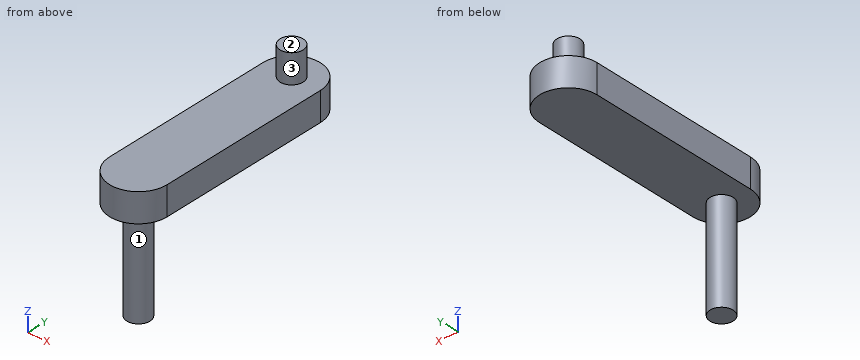
```python
from build123d import *

# Parameters (mm, degrees)
SKETCH1_R           = 4
BOSS_EXTRUDE1_DEPTH = 10
SKETCH1_2_R         = 4
BOSS_EXTRUDE2_DEPTH = 20
BOSS_EXTRUDE3_START = -35
SKETCH1_3_R         = 4
BOSS_EXTRUDE3_DEPTH = 45


with BuildPart() as part:
    # Sketch1 → Boss-Extrude1 (new body)
    with BuildSketch(Plane.XY):
        with BuildLine():
            Line((10, 30), (10, -30))
            ThreePointArc((10, -30), (0, -40), (-10, -30))
            Line((-10, -30), (-10, 30))
            ThreePointArc((-10, 30), (0, 40), (10, 30))
        make_face()
        with Locations((0, 30)):
            Circle(SKETCH1_R, mode=Mode.SUBTRACT)
        with Locations((0, -30)):
            Circle(SKETCH1_R, mode=Mode.SUBTRACT)
    extrude(amount=BOSS_EXTRUDE1_DEPTH)

    # Sketch1<2> → Boss-Extrude2 (add)
    with BuildSketch(Plane.XY):
        with Locations((0, 30)):
            Circle(SKETCH1_2_R)
    extrude(amount=BOSS_EXTRUDE2_DEPTH)

    # Sketch1<3> → Boss-Extrude3 (add)
    with BuildSketch(Plane.XY.offset(BOSS_EXTRUDE3_START)):
        with Locations((0, -30)):
            Circle(SKETCH1_3_R)
    extrude(amount=BOSS_EXTRUDE3_DEPTH)


solid = part.part
```
Geometry: final body of the model. Coordinates: model frame, mm. Face numbers are marked on the shaded views. A direction names the side the tool comes from. Coordinates: 2 decimals unless noted, no trailing zeros. Order: outer loops, then holes, each group sorted by start corner. A loop starts at its lowest first (then second) coordinate and runs counter-clockwise, first axis right, second up. Notation, with made-up numbers: M -3.5,-36 L 19.5,-36 A19 ccw 19.5,-14 Z; hole C 84.5,-33.75 d11. An arc over 180 degrees is marked long. Answer in a Markdown table with one row per item. Add a question column.
Q1. Section query A-A on x = 0. Return the cut outline in (y, z).
Q2. Line query: L1, parallel to Z at x = -2.75, y = -15.5; L2, parallel to Y at x = -0.25, z = -31.5; L3, parallel to X at y = -32, z = -16. Output: solid intervals per line, ascending.
Q3. Section query B-B on z = 14. Return the cut outline in (x, y).
Q4. Section query C-C on y = -13.5. Return the cut outline in (x, z), and give its area (3 significant figures).
Q5. Section query D-D on z = 3. Return the cut outline in (x, y).
Q6. Reachability of the marked faces 1, 2 and 3 from +Z, -Z, +X, -X, +Y, -Y: full face, straight path, thin tool, end or side. Return the list, or none.
Q7. Contact query for flat-ended pins moving along their axis: P1, Ø6, axis at x = 5, y = 10.5, coming from the +Z side; P2, Ø6, axis at x = 3.5, z = -19.5, coming from the +Y side; P3, Ø12, axis at x = 6.5, y = -12, coming from the -Z side. Output: stop coordinate, or through.
Completed:
| question | item | result |
|---|---|---|
| 1 | outline | M -40,0 L -34,0 L -34,-35 L -26,-35 L -26,0 L 40,0 L 40,10 L 34,10 L 34,20 L 26,20 L 26,10 L -40,10 Z |
| 2 | L1 | z = 0 to 10 |
| 2 | L2 | y = -33.99 to -26.01 |
| 2 | L3 | x = -3.46 to 3.46 |
| 3 | outline | C 0,30 d8 |
| 4 | outline | M -10,0 L 10,0 L 10,10 L -10,10 Z |
| 4 | area | 200 mm2 |
| 5 | outline | M -10,-30 A10 ccw 10,-30 L 10,30 A10 ccw -10,30 Z |
| 6 | face 1 | -Z |
| 6 | face 2 | +Z, +X, -X, +Y, -Y |
| 6 | face 3 | +Z |
| 7 | P1 | stops at z = 10 |
| 7 | P2 | stops at y = -26.03 |
| 7 | P3 | stops at z = 0 |
